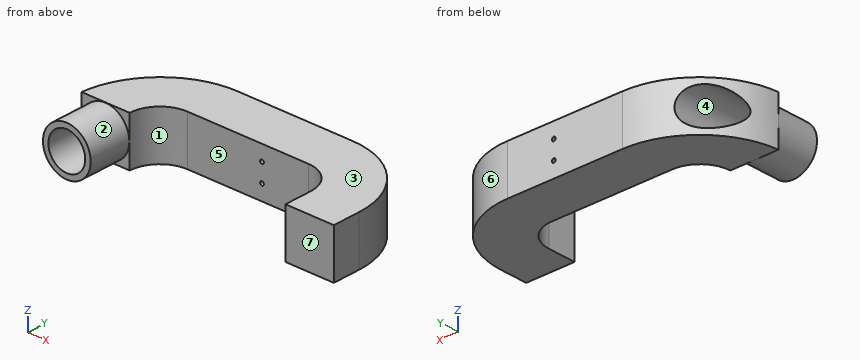
```python
from build123d import *

# Parameters (mm, degrees)
BOSS_EXTRUDE1_DEPTH     = 80
SKETCH5_R               = 59.5
SKETCH5_R_2             = 39.5
CUT_EXTRUDE_THIN2_DEPTH = 70
SKETCH6_R               = 30.5
CUT_EXTRUDE9_DEPTH      = 508.937003968
F_3_0MM_DOWEL_HOLE1_D   = 6.3


with BuildPart() as part:
    # Sketch1 → Boss-Extrude1 (new body)
    with BuildSketch(Plane.XY):
        with BuildLine():
            Line((0, 0), (80, 0))
            Line((80, 0), (80, 70))
            ThreePointArc((80, 70), (94.644660941, 105.355339059), (130, 120))
            Line((130, 120), (235, 120))
            Line((235, 120), (330, 120))
            ThreePointArc((330, 120), (365.355339059, 105.355339059), (380, 70))
            Line((380, 70), (380, 24))
            Line((380, 24), (460, 24))
            Line((460, 24), (460, 70))
            ThreePointArc((460, 70), (421.923881554, 161.923881554), (330, 200))
            Line((330, 200), (140, 200))
            ThreePointArc((140, 200), (41.005050634, 158.994949366), (0, 60))
            Line((0, 60), (0, 0))
        make_face()
    extrude(amount=BOSS_EXTRUDE1_DEPTH)

    # Sketch5 → Cut-Extrude-Thin2 (cut)
    with BuildSketch(Plane.XZ):
        with Locations((40, 40)):
            Circle(SKETCH5_R)
        with Locations((40, 40)):
            Circle(SKETCH5_R_2, mode=Mode.SUBTRACT)
    extrude(amount=-CUT_EXTRUDE_THIN2_DEPTH, mode=Mode.SUBTRACT)

    # Sketch6 → Cut-Extrude9 (cut, through all)
    with BuildSketch(Plane.XZ):
        with Locations(Location((40, 40, 0), (0, 0, 270))):
            Circle(SKETCH6_R)
    extrude(amount=-CUT_EXTRUDE9_DEPTH, mode=Mode.SUBTRACT)

    # Ø3.0mm Dowel Hole1 (through all)
    with Locations(Plane(origin=(253.35, 200, 55), x_dir=(0, 0, 1), z_dir=(0, 1, 0))):
        with Locations((0, 0), (-30, 0)):
            Hole(F_3_0MM_DOWEL_HOLE1_D / 2)


solid = part.part
```
Geometry: final body of the model. Coordinates: model frame, mm. Face numbers are marked on the shaded views. A direction names the side the tool comes from. Give positions to 0.01 mm unless a question says otherwise; leave off trailing zeros. Order: outer loops, then holes, each group sorted by start corner. A loop starts at its lowest first (then second) coordinate and runs counter-clockwise, first axis right, second up. Notation, with made-up numbers: M 54.25,35.5 L 105.25,35.5 A24 ccw 105.25,74.5 Z; hole C -19.75,-14.5 d5. An arc over 180 degrees is marked long. Answer as CSV lines item,"result". Start each with the question number.
1) Line query: line 1 (Z direction, x = 253, y = 167); line 2 (X direction, y = 103, z = 63); line 3 (X direction, y = 93, z = 36.5). Output: solid intervals per line, ascending. Write a range as from..to.
2) First-contact query: P1, Ø1, axis at y = 45.5, z = 52, coming from the -X side; P2, Ø8, axis at y = 137.5, z = 35, coming from the -X side; P3, Ø12, axis at x = 68.5, y = 32, coming from the +Z side. Flat tips, straight axial feed; report the tip coordinate or a pass-through.
3) Mould query, pull axis Z, two halves, no side actions, for the marked faces 1, 2, 3 and 4. Classes: +Z half, -Z half, draft (parallel to the pull), parting line (faces both ways), or undercut.
4) Cut plane A-A (y = 40.5). Output: boundary loops of the cut face in (x, z), then the cut area to 3 significant figures.
5) Cut plane D-D (y = 127.5). Output: boundary loops of the cut face in (x, z).
6) Cut plane C-C (z = 40). Output: boundary loops of the cut face in (x, y).
7) Cut plane B-B (x = 40). Output: boundary loops of the cut face in (y, z), then the cut area to 3 significant figures.
8) Set-up query: the marked faces 5, 6 and 7. Return all of +Z, -Z, +X, -X, +Y, -Y with unobstructed straight access to the full face (end or side cutting, diameter ignored); none if empty.
Findings below:
1,line 1,"z = 0..21.87, 28.13..51.87, 58.13..80"
1,line 2,"x = 6.77..19.97, 60.03..92.44, 367.56..455.74"
1,line 3,"x = 3.94..9.7, 70.3..85.6, 374.4..457.95"
2,P1,"stops at x = 2.21"
2,P2,"stops at x = 69.14"
2,P3,"stops at z = 72.47"
3,face 1,"draft"
3,face 2,"parting line"
3,face 3,"+Z half"
3,face 4,"undercut"
4,outline,"C 40,40 d79; M 380,0 L 460,0 L 460,80 L 380,80 Z; hole C 40,40 d61"
4,area,"8,380 mm²"
5,outline,"M 17.35,0 L 446.59,0 L 446.59,80 L 17.35,80 L 17.35,60.42 A30.5 cw long 17.35,19.58 Z; hole C 253.35,25 d6.3; hole C 253.35,55 d6.3"
6,outline,"M 0.36,70 L 0.5,70 L 0.5,0 L 9.5,0 L 9.5,110.69 A140 ccw Z; M 70.5,0 L 79.5,0 L 79.5,70 L 80,70 A50 cw 130,120 L 330,120 A50 cw 380,70 L 380,24 L 460,24 L 460,70 A130 ccw 330,200 L 140,200 A140 ccw 70.5,181.53 Z"
7,outline,"M 0,0.5 L 70,0.5 L 70,0 L 157.98,0 L 157.98,9.5 L 0,9.5 Z; M 0,70.5 L 157.98,70.5 L 157.98,80 L 70,80 L 70,79.5 L 0,79.5 Z"
7,area,"2,930 mm²"
8,face 5,"+Z, -Z, -Y"
8,face 6,"+Z, -Z, +X, +Y"
8,face 7,"+Z, -Z, +X, -Y"
